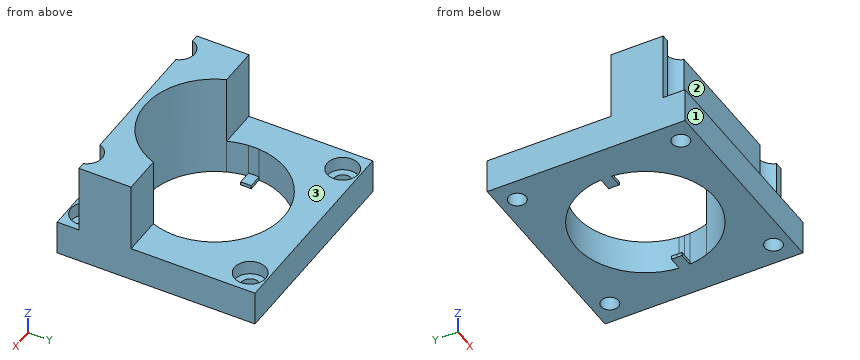
```python
from build123d import *

# Parameters (mm, degrees)
F0_R     = 4.5
F1_DEPTH = 10
F2_DEPTH = 30
F3_DEPTH = 10
F0_R_2   = 2.5
F4_DEPTH = 6
F5_DEPTH = 6
F6_DEPTH = 6
F7_DEPTH = 1


with BuildPart() as f1:
    # F0 (on Top) → F1 (new body)
    with BuildSketch(Plane.XY):
        with BuildLine():
            Line((0, 57), (0, 21.3))
            Line((0, 21.3), (11.302673988, 21.3))
            ThreePointArc((11.302673988, 21.3), (10.4807134754, 24.0413931616), (10.0584521038, 26.8720381207))
            ThreePointArc((10.0584521038, 26.8720381207), (10, 28.4), (10.0584521038, 29.9279618793))
            ThreePointArc((10.0584521038, 29.9279618793), (30, 48.4), (49.9415478962, 29.9279618793))
            ThreePointArc((49.9415478962, 29.9279618793), (49.9853816316, 29.1645397558), (50, 28.4))
            ThreePointArc((50, 28.4), (49.9853816316, 27.6354602442), (49.9415478962, 26.8720381207))
            ThreePointArc((49.9415478962, 26.8720381207), (49.5192865246, 24.0413931616), (48.697326012, 21.3))
            Line((48.697326012, 21.3), (60, 21.3))
            Line((60, 21.3), (60, 57))
            Line((60, 57), (0, 57))
        make_face()
        with Locations((6.4448192716, 51.97)):
            Circle(F0_R, mode=Mode.SUBTRACT)
        with Locations((53.5848192716, 51.97)):
            Circle(F0_R, mode=Mode.SUBTRACT)
    extrude(amount=F1_DEPTH)

    # F0 (on Top) → F2 (join)
    with BuildSketch(Plane.XY):
        with BuildLine():
            Line((0, 21.3), (0, 6.3))
            Line((0, 6.3), (2.1916910111, 6.3))
            ThreePointArc((2.1916910111, 6.3), (6.4448192716, 9.33), (10.697947532, 6.3))
            Line((10.697947532, 6.3), (49.3316910111, 6.3))
            ThreePointArc((49.3316910111, 6.3), (53.5848192716, 9.33), (57.837947532, 6.3))
            Line((57.837947532, 6.3), (60, 6.3))
            Line((60, 6.3), (60, 21.3))
            Line((60, 21.3), (48.697326012, 21.3))
            ThreePointArc((48.697326012, 21.3), (30, 8.4), (11.302673988, 21.3))
            Line((11.302673988, 21.3), (0, 21.3))
        make_face()
    extrude(amount=F2_DEPTH)

    # F0 (on Top) → F3 (join)
    with BuildSketch(Plane.XY):
        with BuildLine():
            Line((0, 6.3), (0, 0))
            Line((0, 0), (60, 0))
            Line((60, 0), (60, 6.3))
            Line((60, 6.3), (57.837947532, 6.3))
            ThreePointArc((57.837947532, 6.3), (58.0226721968, 5.5752928377), (58.0848192716, 4.83))
            ThreePointArc((58.0848192716, 4.83), (52.8395264339, 0.3921470748), (49.3316910111, 6.3))
            Line((49.3316910111, 6.3), (10.697947532, 6.3))
            ThreePointArc((10.697947532, 6.3), (10.8826721968, 5.5752928377), (10.9448192716, 4.83))
            ThreePointArc((10.9448192716, 4.83), (5.6995264339, 0.3921470748), (2.1916910111, 6.3))
            Line((2.1916910111, 6.3), (0, 6.3))
        make_face()
    extrude(amount=F3_DEPTH)

    # F0 (on Top) → F4 (join)
    with BuildSketch(Plane.XY):
        with BuildLine():
            ThreePointArc((10.697947532, 6.3), (6.4448192716, 9.33), (2.1916910111, 6.3))
            ThreePointArc((2.1916910111, 6.3), (5.6995264339, 0.3921470748), (10.9448192716, 4.83))
            ThreePointArc((10.9448192716, 4.83), (10.8826721968, 5.5752928377), (10.697947532, 6.3))
        make_face()
        with Locations((6.4448192716, 4.83)):
            Circle(F0_R_2, mode=Mode.SUBTRACT)
    extrude(amount=F4_DEPTH)

    # F0 (on Top) → F5 (join)
    with BuildSketch(Plane.XY):
        with BuildLine():
            ThreePointArc((58.0848192716, 4.83), (58.0226721968, 5.5752928377), (57.837947532, 6.3))
            ThreePointArc((57.837947532, 6.3), (53.5848192716, 9.33), (49.3316910111, 6.3))
            ThreePointArc((49.3316910111, 6.3), (52.8395264339, 0.3921470748), (58.0848192716, 4.83))
        make_face()
        with Locations((53.5848192716, 4.83)):
            Circle(F0_R_2, mode=Mode.SUBTRACT)
    extrude(amount=F5_DEPTH)

    # F0 (on Top) → F6 (join)
    with BuildSketch(Plane.XY):
        with Locations((6.4448192716, 51.97)):
            Circle(F0_R)
        with Locations((6.4448192716, 51.97)):
            Circle(F0_R_2, mode=Mode.SUBTRACT)
        with Locations((53.5848192716, 51.97)):
            Circle(F0_R)
        with Locations((53.5848192716, 51.97)):
            Circle(F0_R_2, mode=Mode.SUBTRACT)
    extrude(amount=F6_DEPTH)

    # F0 (on Top) → F7 (join)
    with BuildSketch(Plane.XY):
        with BuildLine():
            ThreePointArc((10.0584521038, 29.9279618793), (10, 28.4), (10.0584521038, 26.8720381207))
            Line((10.0584521038, 26.8720381207), (14.0731254637, 26.8720381207))
            ThreePointArc((14.0731254637, 26.8720381207), (14, 28.4), (14.0731254637, 29.9279618793))
            Line((14.0731254637, 29.9279618793), (10.0584521038, 29.9279618793))
        make_face()
        with BuildLine():
            Line((45.9268745363, 26.8720381207), (49.9415478962, 26.8720381207))
            ThreePointArc((49.9415478962, 26.8720381207), (49.9853816316, 27.6354602442), (50, 28.4))
            ThreePointArc((50, 28.4), (49.9853816316, 29.1645397558), (49.9415478962, 29.9279618793))
            Line((49.9415478962, 29.9279618793), (45.9268745363, 29.9279618793))
            ThreePointArc((45.9268745363, 29.9279618793), (45.9817081781, 29.164855352), (46, 28.4))
            ThreePointArc((46, 28.4), (45.9817081781, 27.635144648), (45.9268745363, 26.8720381207))
        make_face()
    extrude(amount=F7_DEPTH)


solid = f1.part
```
Verification items for the finished model (mm, model axes). Face numbers are marked on the shaded views. A direction names the side the tool comes from. Give positions to 0.01 mm unless a question says otherwise; leave off trailing zeros. Loops run counter-clockwise (first coordinate to the right, second up) from the corner with the lowest first, then second, coordinate; pieces in that order, holes last. Notation, with made-up numbers: M 88,-3.5 L 135,-3.5 A31 ccw 135,25.5 Z; hole C 65.25,-12.75 d4. An arc over 180 degrees is marked long. One line per question, with ' | ' between items.
Item 1: Depth check by flat-ended pin: P1, Ø2, axis at y = 15, z = 17.5, coming from the -X side; P2, Ø3.5, axis at x = 47, y = 28, coming from the +Z side; P3, Ø4.5, axis at x = 6, y = 4, coming from the +Z side; P4, Ø1.1, axis at x = 59, z = 19, coming from the -Y side. Enter the tip coordinate at first touch or a pass-through.
Completed:
P1: stops at x = 0 | P2: stops at z = 1 | P3: stops at z = 6 | P4: stops at y = 6.3
Item 2: Thickness scan on line 1 (X direction, y = 4.83, z = 8.95); line 2 (X direction, y = 7.5, z = 20.75); line 3 (Y direction, x = 57, z = 8). Record the ranges inside material, lowest first. Write a range as [from, to].
Completed:
line 1: x = [0, 1.94], [10.94, 49.08], [58.08, 60] | line 2: x = [0, 2.82], [10.07, 49.96], [57.21, 60] | line 3: y = [0, 1.9], [7.76, 49.04], [54.9, 57]
Item 3: Section check D-D, the plane x = 33. Record the cut outline in (y, z), plus the area to 3 significant figures.
Completed:
outline: M 0,0 L 8.63,0 L 8.63,30 L 6.3,30 L 6.3,10 L 0,10 Z; M 48.17,0 L 57,0 L 57,10 L 48.17,10 Z | area: 221 mm^2
Item 4: Section check A-A, the plane y = 24. Record the cut outline in (x, z).
Completed:
outline: M 0,0 L 10.49,0 L 10.49,10 L 0,10 Z; M 49.51,0 L 60,0 L 60,10 L 49.51,10 Z
Item 5: Section check C-C, the plane x = 13. Record the cut outline in (y, z), plus the area to 3 significant figures.
Completed:
outline: M 0,0 L 17.86,0 L 17.86,30 L 6.3,30 L 6.3,10 L 0,10 Z; M 26.87,0 L 29.93,0 L 29.93,1 L 26.87,1 Z; M 38.94,0 L 57,0 L 57,10 L 38.94,10 Z | area: 594 mm^2
Item 6: Section check B-B, the plane y = 51.97. Record the cut outline in (x, z), plus the area to 3 significant figures.
Completed:
outline: M 0,0 L 3.94,0 L 3.94,6 L 1.94,6 L 1.94,10 L 0,10 Z; M 8.94,0 L 51.08,0 L 51.08,6 L 49.08,6 L 49.08,10 L 10.94,10 L 10.94,6 L 8.94,6 Z; M 56.08,0 L 60,0 L 60,10 L 58.08,10 L 58.08,6 L 56.08,6 Z | area: 468 mm^2
Item 7: Tool access check on the marked faces 1, 2 and 3. Record the directions out of +Z, -Z, +X, -X, +Y, -Y that give a thin tool (end or side, any length) a straight path to the whole face; none if there is none.
Completed:
face 1: +Z, -Z, +X, -X, -Y | face 2: +Z, +X, -X, -Y | face 3: +Z, +X, -X, +Y
